Input: part model. Units: mm. Frame: model coordinates. Round coordinates to 2 decimals unless told otherwise and drop trailing zeros. Order: outer loops, then holes, each group sorted by start corner. A loop starts at its lowest first (then second) coordinate and runs counter-clockwise, first axis right, second up. Notation, with made-up numbers: M 3.5,82 L 46.5,82 A15 ccw 46.5,91 Z; hole C 6,9.5 d1. An arc over 180 degrees is marked long. One line per question, with ' | ' between items.
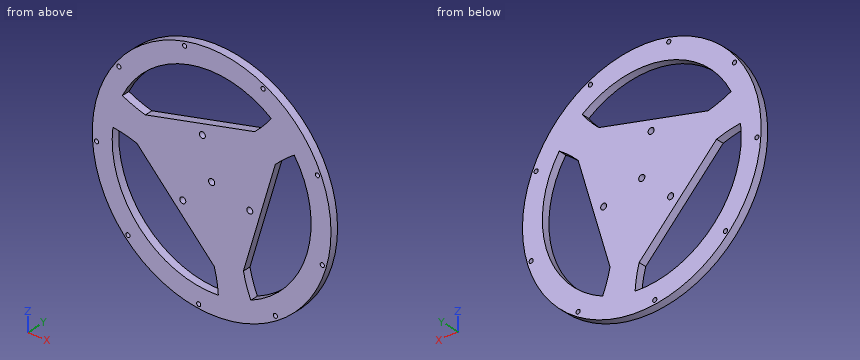
```python
from build123d import *

# Parameters (mm, degrees)
SKETCH_3_R           = 60
SKETCH_3_R_2         = 1.052935028
SKETCH_3_R_3         = 1.5
EXTRUDE_4_DEPTH      = 4
CUT_EXTRUDE_15_DEPTH = 4
SKETCH_3_22_R        = 1.55
CUT_EXTRUDE_23_DEPTH = 10
SKETCH_3_23_R        = 1.052935028
CUT_EXTRUDE_24_DEPTH = 10


with BuildPart() as part:
    # 草图3 → 凸台-拉伸4 (new body)
    with BuildSketch(Plane(origin=(0, 0, 0), x_dir=(1, 0, 0), z_dir=(0, 1, 0))):
        Circle(SKETCH_3_R)
        with Locations((-46.641583195, -34.475537952)):
            Circle(SKETCH_3_R_2, mode=Mode.SUBTRACT)
        with Locations((-13.569076992, -56.390426045)):
            Circle(SKETCH_3_R_2, mode=Mode.SUBTRACT)
        with BuildLine():
            ThreePointArc((-44.889569885, -22.021047103), (-39.209954392, -19.560908928), (-33.307112163, -17.698983687))
            Line((-33.307112163, -17.698983687), (21.609631998, -30.913452559))
            ThreePointArc((21.609631998, -30.913452559), (26.019303967, -35.256850436), (29.958048994, -40.031428909))
            ThreePointArc((29.958048994, -40.031428909), (-11.697480165, -48.612436246), (-44.889569885, -22.021047103))
        make_face(mode=Mode.SUBTRACT)
        with Locations((-4.678992066, -19.444974498)):
            Circle(SKETCH_3_R_3, mode=Mode.SUBTRACT)
        with Locations((25.852551139, -51.919607083)):
            Circle(SKETCH_3_R_2, mode=Mode.SUBTRACT)
        with Locations((53.177483273, -23.155026944)):
            Circle(SKETCH_3_R_2, mode=Mode.SUBTRACT)
        with Locations((-14.500345858, 13.774613243)):
            Circle(SKETCH_3_R_3, mode=Mode.SUBTRACT)
        with BuildLine():
            ThreePointArc((15.967019236, 34.171216556), (17.523676152, 40.161803442), (19.689209887, 45.960145931))
            ThreePointArc((19.689209887, 45.960145931), (47.948344812, 14.175903139), (41.515571152, -27.864984334))
            ThreePointArc((41.515571152, -27.864984334), (36.545221249, -24.176362121), (31.981325576, -19.995313417))
            Line((31.981325576, -19.995313417), (15.967019236, 34.171216556))
        make_face(mode=Mode.SUBTRACT)
        with Locations((55.620079982, 16.444047642)):
            Circle(SKETCH_3_R_2, mode=Mode.SUBTRACT)
        with Locations((32.037423118, 48.34876958)):
            Circle(SKETCH_3_R_2, mode=Mode.SUBTRACT)
        with Locations((-42.05100299, 39.946378404)):
            Circle(SKETCH_3_R_2, mode=Mode.SUBTRACT)
        with Locations((-6.535900078, 57.630564895)):
            Circle(SKETCH_3_R_2, mode=Mode.SUBTRACT)
        with Locations((19.179337925, 5.670361256)):
            Circle(SKETCH_3_R_3, mode=Mode.SUBTRACT)
    extrude(amount=EXTRUDE_4_DEPTH)

    # 草图3<17> → 切除-拉伸15 (cut)
    with BuildSketch(Plane(origin=(0, 0, 0), x_dir=(1, 0, 0), z_dir=(0, 1, 0))):
        with BuildLine():
            Line((1.325786588, 37.694297104), (-37.576651234, -3.257763997))
            ThreePointArc((-37.576651234, -3.257763997), (-43.542980118, -4.904953006), (-49.647258882, -5.928717023))
            ThreePointArc((-49.647258882, -5.928717023), (-36.250864646, 34.436533107), (3.373998733, 49.886031437))
            ThreePointArc((3.373998733, 49.886031437), (2.664733143, 43.737271049), (1.325786588, 37.694297104))
        make_face()
    extrude(amount=CUT_EXTRUDE_15_DEPTH, mode=Mode.SUBTRACT)

    # 草图3<22> → 切除-拉伸23 (cut)
    with BuildSketch(Plane(origin=(0, 0, 0), x_dir=(1, 0, 0), z_dir=(0, 1, 0))):
        Circle(SKETCH_3_22_R)
    extrude(amount=CUT_EXTRUDE_23_DEPTH, mode=Mode.SUBTRACT)

    # 草图3<23> → 切除-拉伸24 (cut)
    with BuildSketch(Plane(origin=(0, 0, 0), x_dir=(1, 0, 0), z_dir=(0, 1, 0))):
        with Locations((-57.889974257, 3.570837502)):
            Circle(SKETCH_3_23_R)
    extrude(amount=CUT_EXTRUDE_24_DEPTH, mode=Mode.SUBTRACT)


solid = part.part
```
Item 1: Section query D-D, the plane y = 2.3. Give the number of separate pieces and of enclosed holes in the cut face, plus the area to 3 significant figures.
Report:
separate pieces: 1 | enclosed holes: 16 | area: 6,950 mm²
Item 2: Line query: line 1 along Z through (x, y) = (32.5, 2.35); line 2 along Z through (x, y) = (-4.5, 2.2); line 3 along X through (y, z) = (1.95, -16). Output: solid intervals per line, ascending. Write a range as from..to.
Report:
line 1: -50.44..-49.29, -47.4..-38, 20.52..50.44 | line 2: -59.83..-49.8, -31.56..17.96, 20.93..24.63, 49.8..59.83 | line 3: -57.83..-47.37, -19.28..21.34, 47.37..54.67, 56.57..57.83
Item 3: Section query C-C, the plane z = -30.5. Return loops of the section in (x, y), plus the area to 3 significant figures.
Report:
outline: M -51.67,0 L -39.62,0 L -39.62,4 L -51.67,4 Z; M -5.51,0 L 17.05,0 L 17.05,4 L -5.51,4 Z; M 39.62,0 L 51.67,0 L 51.67,4 L 39.62,4 Z | area: 187 mm²
Item 4: Section query A-A, the plane x = 38.5. Return loops of the section in (y, z), plus the area to 3 significant figures.
Report:
outline: M 0,-46.02 L 4,-46.02 L 4,-31.9 L 0,-31.9 Z; M 0,25.72 L 4,25.72 L 4,46.02 L 0,46.02 Z | area: 138 mm²
Item 5: First-contact query: pin 1 (2.5 mm diameter, centred on x = -13.57, z = 56.39, fed in from +Y); pin 2 (2 mm diameter, centred on y = 2, z = 8.5, fed in from +X); pin 3 (1 mm diameter, centred on y = 2, z = -20.5, fed in from -X); pin 4 (1.5 mm diameter, centred on x = 28, y = 3.5, fed in from -Z) (3 decimals). Flat tips, straight axial feed; report the tip coordinate or a pass-through.
Report:
pin 1: y = 4 | pin 2: x = 59.53 | pin 3: x = -56.57 | pin 4: z = -53.455
Item 6: Section query B-B, the plane z = 0. Return loops of the section in (x, y).
Report:
outline: M -60,0 L -50,0 L -50,4 L -60,4 Z; M -34.48,0 L -1.55,0 L -1.55,4 L -34.48,4 Z; M 1.55,0 L 26.07,0 L 26.07,4 L 1.55,4 Z; M 50,0 L 60,0 L 60,4 L 50,4 Z
